from build123d import *

# Parameters (mm, degrees)
BOSS_EXTRUDE1_DEPTH      = 30.956
BOSS_EXTRUDE1_DEPTH_BACK = 2
CUT_EXTRUDE1_DEPTH       = 50.013690395
CUT_EXTRUDE1_DEPTH_BACK  = 50.013690395


with BuildPart() as part:
    # Sketch1 → Boss-Extrude1 (new, two sides: drawn at the far end of the back side and taken through both)
    with BuildSketch(Plane.XY.offset(-BOSS_EXTRUDE1_DEPTH_BACK)):
        with BuildLine():
            Line((-3.6, 36.195), (-3.6, -5.427367667))
            ThreePointArc((-3.6, -5.427367667), (3.9877, -13.015067667), (11.5754, -5.427367667))
            Line((11.5754, -5.427367667), (11.5754, 16.475329119))
            Line((11.5754, 16.475329119), (0.976429971, 36.195))
            Line((0.976429971, 36.195), (-3.6, 36.195))
        make_face()
    extrude(amount=BOSS_EXTRUDE1_DEPTH + BOSS_EXTRUDE1_DEPTH_BACK)

    # Sketch2 → Cut-Extrude1 (cut, two sides: drawn at the far end of the back side and taken through both)
    with BuildSketch(Plane.ZY.offset(-CUT_EXTRUDE1_DEPTH_BACK)):
        Polygon((-2, 29.667962996), (7.4890837, 36.195), (21.4669163, 36.195), (30.956, 29.667962996), (30.956, 40.573926282), (-2, 40.573926282), align=None)
        Polygon((-6.302377798, -4.81069075), (9.259609163, -17.017997888), (16.714453216, -17.017997888), (37.494831014, -3.133350838), (37.494831014, -21.39692417), (-6.302377798, -21.39692417), align=None)
    extrude(amount=CUT_EXTRUDE1_DEPTH + CUT_EXTRUDE1_DEPTH_BACK, mode=Mode.SUBTRACT)


solid = part.part
The listing builds one solid part. Answer for the finished solid, in the listing's coordinates (mm). Round coordinates to 2 decimals unless told otherwise and drop trailing zeros. Write each loop counter-clockwise with the first axis right and the second up, starting at its lowest first coordinate (ties: lowest second). Pieces come first, ordered by that corner, then holes. Notation, with made-up numbers: M 50.5,33.25 L 105.5,33.25 A14 cw 105.5,47.25 Z; hole C 71.5,75.25 d11. An arc over 180 degrees is marked long. Write each question's results on one line, items separated by ' | '. Start each with the question number.
Item 1: Straight lines are drawn through the part: probe 1 along Y at (x, z) = (-0.75, 19) (3 decimals); probe 2 along Y at (x, z) = (7.25, 16); probe 3 along X at (y, z) = (23.5, 22). For each, find the intervals that lie inside material, in ascending order.
Item 2: Find section C-C on y = 18.5. Write down the section's boundary in (x, z).
Item 3: Find section A-A on z = 14. Write down the section's boundary in (x, y) (3 decimals), and give its area (3 significant figures).
Item 4: Find section B-B on x = -1.25. Write down the section's boundary in (y, z) (3 decimals), and give its area (3 significant figures).
Item 5: Given pin 1 Ø1 at (x, z) = (7, 26.5) entering from +Y; pin 2 Ø12 at (y, z) = (30.5, 9.5) entering from +X; pin 3 Ø10 at (y, z) = (21.5, 19.5) entering from +X, each flat-ended and moving along its own axis, determine where each tip first touches the part or whether it passes through.
Item 6: Find section D-D on x = 2.5. Write down the section's boundary in (y, z).
Answer block:
1) probe 1: y = -11.354 to 36.195 | probe 2: y = -12.28 to 24.52 | probe 3: x = -3.6 to 7.8
2) outline: M -3.6,-2 L 10.49,-2 L 10.49,30.96 L -3.6,30.96 Z
3) outline: M -3.6,-5.427 A7.588 ccw 11.575,-5.427 L 11.575,16.475 L 0.976,36.195 L -3.6,36.195 Z | area: 618 mm²
4) outline: M -10.917,1.482 L -8.186,-2 L 29.668,-2 L 36.195,7.489 L 36.195,21.467 L 29.668,30.956 L -7.502,30.956 L -10.917,25.845 Z | area: 1,480 mm²
5) pin 1: stops at y = 25.92 | pin 2: stops at x = 7.26 | pin 3: stops at x = 11.56
6) outline: M -12.87,3.97 L -8.19,-2 L 29.67,-2 L 33.36,3.37 L 33.36,25.59 L 29.67,30.96 L -7.5,30.96 L -12.87,22.93 Z
